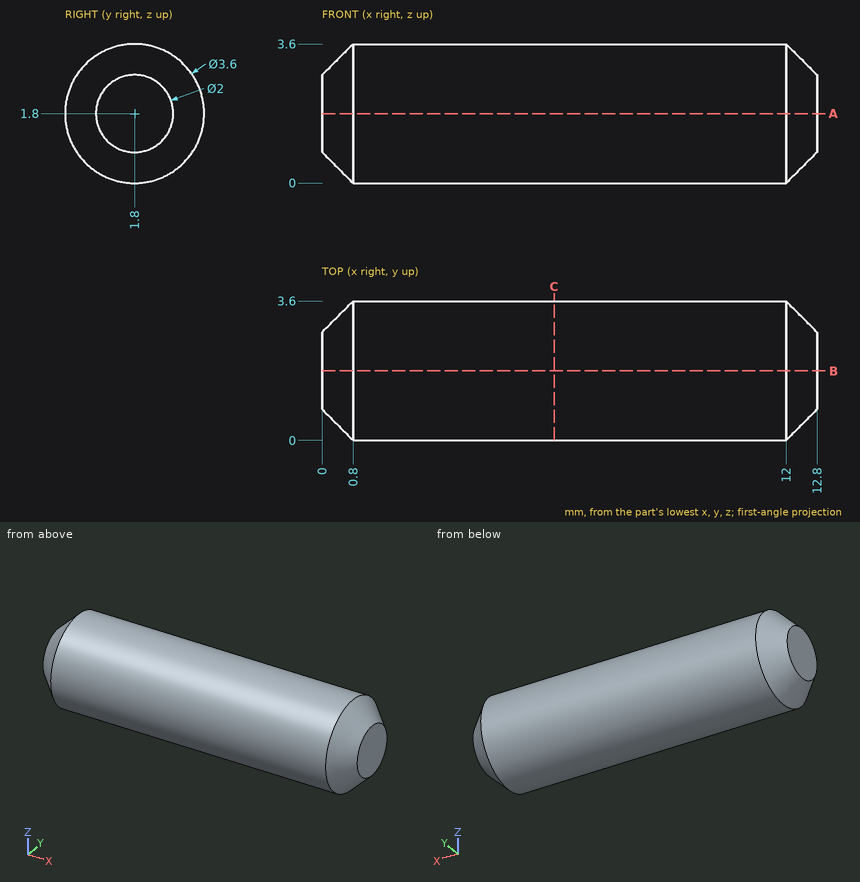
Design review of the part shown in the three views and the two pictorial views. Dimensions are in mm from the part's minimum x, y and z. Coordinates: 2 decimals unless noted, no trailing zeros. Order: outer loops, then holes, each group sorted by start corner. A loop starts at its lowest first (then second) coordinate and runs counter-clockwise, first axis right, second up. Notation, with made-up numbers: (32, 63.25) - (41, 63.25) arc R24 ccw to (41, 99.25) - close; hole circle Ø3 at (-4, -20). An arc over 180 degrees is marked (long way). Answer as CSV lines item,"result". Start each with the question number.
1) To check wall thickness, follow line 1 along Z through (x, y) = (8, 0.6); line 2 along Z through (x, y) = (5, 1.55); line 3 along Y through (x, z) = (10.75, 1.3). State the ranges of each line that lie inside material, in increasing order. Write a range as [from, to].
2) Add section A-A (z = 1.8). State the section outline as (x, y) points.
3) Add section C-C (x = 6). State the section outline as (y, z) points, then the cut area to 3 significant figures.
Result:
1,line 1,"[0.46, 3.14]"
1,line 2,"[0.02, 3.58]"
1,line 3,"[0.07, 3.53]"
2,outline,"(0, 0.8) - (0.8, 0) - (12, 0) - (12.8, 0.8) - (12.8, 2.8) - (12, 3.6) - (0.8, 3.6) - (0, 2.8) - close"
3,outline,"circle Ø3.6 at (1.8, 1.8)"
3,area,"10.2 mm^2"
